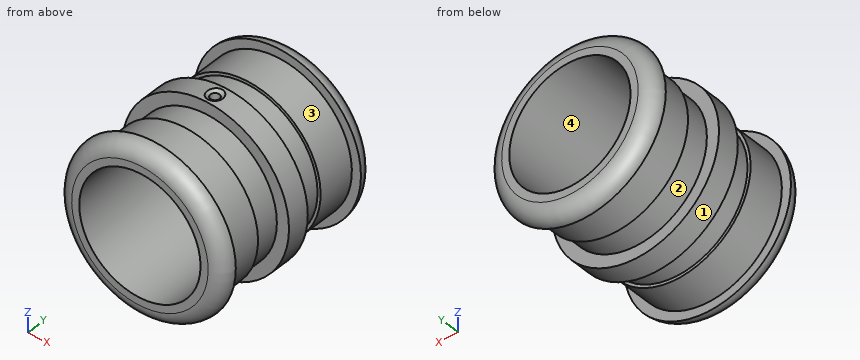
from build123d import *

# Parameters (mm, degrees)
F4_R = 9.99999


# Not quite as in the source:
# - a fillet or chamfer is up to 0.001 mm smaller than in the source, because OpenCascade refuses the exact size


with BuildPart() as f1:
    # F0 (on Right) → F1 (revolve)
    with BuildSketch(Plane.YZ):
        Polygon((-60, 55), (-60, 40), (60, 40), (60, 55), (50, 55), (50, 49), (25, 49), (25, 47), (7.5, 47), (7.5, 55), (-7.5, 55), (-7.5, 47), (-25, 47), (-25, 49), (-50, 49), (-50, 55), align=None)
    revolve(axis=Axis((0, -7.7097125049, 0), (0, 1, 0)))

    # F2 (on Right) → F3 (revolve, cut)
    with BuildSketch(Plane.YZ):
        Polygon((7.2320508076, 56), (0, 56), (0, 36), (3, 36), (3, 53.556624327), align=None)
    revolve(axis=Axis((0, 0, 50.0545714922), (0, 0, -1)), mode=Mode.SUBTRACT)

    # F4 (radius 10 in the source; OpenCascade refuses exactly that, so slightly less here)
    f4_edges = [f1.edges().sort_by_distance(p)[0] for p in [
        (0, 60, -55),
        (0, -60, -55),
    ]]
    fillet(f4_edges, radius=F4_R)


solid = f1.part
Can you work these out from the model? Positions are in its coordinate system, mm. Face numbers are marked on the shaded views. A direction names the side the tool comes from. Give positions to 0.01 mm unless a question says otherwise; leave off trailing zeros. Order: outer loops, then holes, each group sorted by start corner. A loop starts at its lowest first (then second) coordinate and runs counter-clockwise, first axis right, second up. Notation, with made-up numbers: M 1,89 L 56,89 A20 cw 56,126 Z; hole C 71.5,-24 d5. An arc over 180 degrees is marked long. Use a Markdown table: item, result. Add a question column.
Item 1: Suppose I cut it at D-D (y = -39.5). List the corners of the cut face in (x, z) for me, then the cut area to 3 significant figures.
Item 2: Suppose I cut it at A-A (y = 23). List the corners of the cut face in (x, z) for me.
Item 3: For the marked faces 1 and 2, which set-ups out of +Z, -Z, +X, -X, +Y, -Y let a thin tool reach every point of the face, with its end or its side?
Item 4: Will these pins go through, and if not, where does the flat tip stop? pin 1 (2 mm diameter, centred on y = 7, z = -42, fed in from +X); pin 2 (12 mm diameter, centred on x = 30.5, z = -0.5, fed in from -Y); pin 3 (5 mm diameter, centred on x = 32.5, y = 31, fed in from +Z); pin 4 (12 mm diameter, centred on y = -15, z = 40.5, fed in from +X).
Item 5: We'd pull the mould along X, two halves only. Please class the marked faces 3 and 4: +X half, -X half, draft (parallel to the pull), parting line (faces both ways), or undercut.
Item 6: Suppose I cut it at B-B (x = 0). Count the separate pieces of the cut face and the enclosed holes in it, then the cut area to 3 significant figures.
Item 7: If I drill on L1, parallel to Y at x = 33.5, z = 42; L2, parallel to Y at x = 0, z = 48; L3, parallel to X at y = 0, z = 49, over which ranges is the centre line in solid material (lowest first)? Write a range as [from, to].
Item 8: Suppose I cut it at C-C (y = 0). List the corners of the cut face in (x, z) for me.
Answer sheet:
| question | item | result |
|---|---|---|
| 1 | outline | C 0,0 d98; hole C 0,0 d80 |
| 1 | area | 2,520 mm² |
| 2 | outline | C 0,0 d94; hole C 0,0 d80 |
| 3 | face 1 | +Y, -Y |
| 3 | face 2 | none |
| 4 | pin 1 | stops at x = 36.66 |
| 4 | pin 2 | passes through |
| 4 | pin 3 | stops at z = 38.74 |
| 4 | pin 4 | stops at x = 31.92 |
| 5 | face 3 | parting line |
| 5 | face 4 | undercut |
| 6 | separate pieces | 3 |
| 6 | enclosed holes | 0 |
| 6 | area | 2,260 mm² |
| 7 | L1 | y = [-54.89, -50], [-7.5, 7.5], [50, 54.89] |
| 7 | L2 | y = [-59.54, -25], [-7.5, -3], [3, 7.5], [25, 59.54] |
| 7 | L3 | x = [-24.98, -3], [3, 24.98] |
| 8 | outline | M -5.09,54.76 A55 ccw long 5.09,54.76 L 3,53.56 L 3,39.89 A40 cw long -3,39.89 L -3,53.56 Z |
